```python
from build123d import *

# Parameters (mm, degrees)
F0_W      = 80
F0_H      = 50
F1_DEPTH  = 30
F2_W      = 50
F2_H      = 45
F3_DEPTH  = 10
F4_W      = 50
F4_H      = 40
F5_DEPTH  = 15
F6_W      = 10
F6_H      = 20
F7_DEPTH  = 15
F11_W     = 98.4419174492
F11_H     = 69.922182709
F12_DEPTH = 30


with BuildPart() as f1:
    # F0 (on Front) → F1 (new body, symmetric)
    with BuildSketch(Plane.XZ):
        Rectangle(F0_W, F0_H)
    extrude(amount=F1_DEPTH, both=True)

    # F2 (on face) → F3 (cut)
    with BuildSketch(Plane.XY.offset(25)):
        with Locations((-5, -7.5)):
            Rectangle(F2_W, F2_H)
    extrude(amount=-F3_DEPTH, mode=Mode.SUBTRACT)

    # F4 (on face) → F5 (cut)
    with BuildSketch(Plane.XZ.offset(30)):
        with Locations((-5, -5)):
            Rectangle(F4_W, F4_H)
    extrude(amount=-F5_DEPTH, mode=Mode.SUBTRACT)

    # F6 (on face) → F7 (cut)
    with BuildSketch(Plane.XZ.offset(30)):
        with Locations((-35, -15)):
            Rectangle(F6_W, F6_H)
    extrude(amount=-F7_DEPTH, mode=Mode.SUBTRACT)

    # F11 (on 3pt) → F12 (cut)
    with BuildSketch(Plane(origin=(4.3831168831, -11.6883116883, 13.1493506494), x_dir=(0.9703393435, 0.1606078913, -0.1806838778), z_dir=(0.2417468892, -0.6446583712, 0.7252406676))):
        with Locations((-5.011850968, -1.6786511987)):
            Rectangle(F11_W, F11_H)
    extrude(amount=F12_DEPTH, mode=Mode.SUBTRACT)


solid = f1.part
```
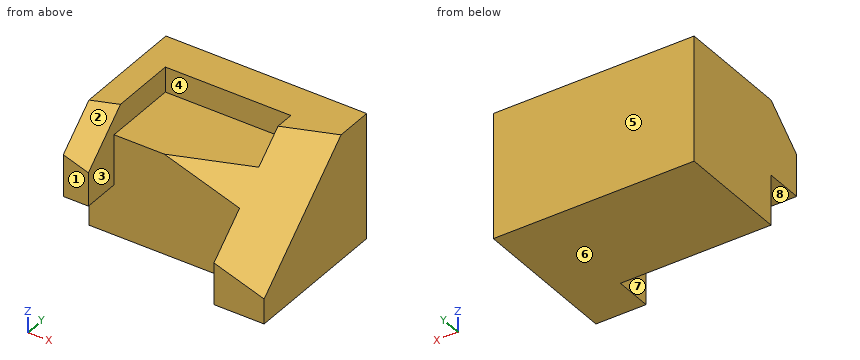
Geometry check sheet. Reference: the model listing, model coordinates, mm. Face numbers are marked on the shaded views. A direction names the side the tool comes from. Give positions to 0.01 mm unless a question says otherwise; leave off trailing zeros. Loops run counter-clockwise (first coordinate to the right, second up) from the corner with the lowest first, then second, coordinate; pieces in that order, holes last. Notation, with made-up numbers: M 73.5,-27 L 119.5,-27 A27 cw 119.5,10 Z; hole C -23,89.25 d11. An arc over 180 degrees is marked long. Answer as CSV lines item,"result".
Item 1: Cross-section at A-A on y = -22. Record the cut outline in (x, z).
Values:
outline,"M -40,-5 L -30,-5 L -30,15.44 L -40,18.78 Z; M 20,-25 L 40,-25 L 40,-7.89 L 20,-1.22 Z"
Item 2: Access from +Z, -Z, +X, -X, +Y, -Y to the whole of each face (thin tool, end or side, straight path). Record for the marked faces 4, 5, 6, 7 and 8.
Values:
face 4,"+Z, -Y"
face 5,"+Z, -Z, +X, -X, +Y"
face 6,"-Z, +X, -X, +Y, -Y"
face 7,"+Z, -Z, -Y"
face 8,"-Z, -X, -Y"
Item 3: Material ranges on line 1 (X direction, y = -26, z = -3); line 2 (Y direction, x = -27, z = -9.5); line 3 (Z direction, x = 7, y = -8.5), recorded low to high.
Values:
line 1,"x = -40 to -30"
line 2,"y = -15 to 30"
line 3,"z = -25 to 15"
Item 4: Cross-section at C-C on z = -16. Record the cut outline in (x, y).
Values:
outline,"M -40,-15 L 20,-15 L 20,-30 L 40,-30 L 40,30 L -40,30 Z"
Item 5: Cross-section at B-B on x = -22. Record the cut outline in (y, z), and give its area (3 significant figures).
Values:
outline,"M -15,-25 L 30,-25 L 30,25 L 15,25 L 15,15 L -15,15 Z"
area,"1,950 mm²"
Item 6: Cross-section at D-D on y = 10.5. Record the cut outline in (x, z), and give its area (3 significant figures).
Values:
outline,"M -40,-25 L 40,-25 L 40,21 L 28,25 L 20,25 L 20,15 L -30,15 L -30,25 L -40,25 Z"
area,"3,480 mm²"
Item 7: Release check for a two-part mould opening along X. For the marked faces 1, 2 and 3 record: pulls with the +X half, pulls with the -X half, needs draft (parallel to the pull), parting line crosses it, or undercut.
Values:
face 1,"needs draft"
face 2,"pulls with the +X half"
face 3,"undercut"
Item 8: Depth check by flat-ended pin: P1, Ø10, axis at x = -7.5, y = 8.5, coming from the +Z side; P2, Ø5, axis at x = -37, y = -25.5, coming from the -Z side; P3, Ø5, axis at x = -13, z = 21, coming from the -Y side; P4, Ø24, axis at y = -4, z = 13, coming from the +X side. Enter the tip coordinate at first touch or a pass-through.
Values:
P1,"stops at z = 15"
P2,"stops at z = -5"
P3,"stops at y = 15"
P4,"stops at x = 40"
